Check sheet for the modelled part. Datum: model origin and axes. Units: mm. A direction names the side the tool comes from. Coordinates: 2 decimals unless noted, no trailing zeros. Write each loop counter-clockwise with the first axis right and the second up, starting at its lowest first coordinate (ties: lowest second). Pieces come first, ordered by that corner, then holes. Notation, with made-up numbers: (-14, 40) - (19, 40) arc R20 ccw to (19, 63) - close; hole circle Ø11 at (57.5, 54.5). An arc over 180 degrees is marked (long way). Use one line per item in the form item = value. Start each with the question number.
1. Draft check along Y on faces 1 (the face through (-49.77, 11.85, -10.54)), 2 (the face through (87.24, 4.95, -10.54)), 3 (the face through (217.75, -5.45, -10.54)). Enter one of: +Y half, -Y half, draft (parallel to the pull), parting line (faces both ways), or undercut.
2. Scan lines: line 1 along Y through (x, z) = (197, -9.5); line 2 along Y through (x, z) = (161, -12.1); line 3 along Y through (x, z) = (126.5, -12.05). Record each from-to range of solid material in increasing order.
3. Cross-section at A-A on z = -12.5. Record the boundary of the cut face in (x, y).
4. Cross-section at C-C on y = -34. Record the boundary of the cut face in (x, z).
5. Cross-section at B-B on x = 173. Record the boundary of the cut face in (y, z), then the cut area to 3 significant figures.
6. Go/stop test with flat-tipped pins: pin 1 Ø1.5 at (x, z) = (13.5, -11) entering from -Y; pin 2 Ø1.5 at (y, z) = (4, -8.5) entering from -X; pin 3 Ø2 at (x, z) = (-4, -12) entering from +Y. Record where each tip stops, or that it passes through.
7. Tool access check on faces 4 (the face through (159, -12.5, -11)), 5 (the face through (237.707, 7.5, -10.542)). Record the directions out of +Z, -Z, +X, -X, +Y, -Y that give a thin tool (end or side, any length) a straight path to the whole face; none if there is none.
```python
from build123d import *

# Parameters (mm, degrees)
SKETCH4_R           = 2.55
SKETCH4_R_2         = 2.549999993
SKETCH4_R_3         = 6
BOSS_EXTRUDE1_DEPTH = 6
CUT_EXTRUDE1_DEPTH  = 10


with BuildPart() as part:
    # Sketch4 → Boss-Extrude1 (new body)
    with BuildSketch(Plane.XY.offset(-13.5)):
        with BuildLine():
            Line((197.399795586, 12.5), (89.263654418, 12.5))
            ThreePointArc((89.263654418, 12.5), (87.876262264, 12.337391799), (86.564070557, 11.858381004))
            ThreePointArc((86.564070557, 11.858381004), (21.105246497, -3.69943352), (-44.353577564, 11.858381004))
            ThreePointArc((-44.353577564, 11.858381004), (-49.84201029, 11.812468541), (-52.996718657, 7.321052632))
            ThreePointArc((-52.996718657, 7.321052632), (-26.920402355, -46.233558559), (32.526685027, -42.476637828))
            ThreePointArc((32.526685027, -42.476637828), (74.2820165, -20.197808109), (120.978886956, -12.5))
            Line((120.978886956, -12.5), (197.399795586, -12.5))
            ThreePointArc((197.399795586, -12.5), (199.721224158, -12.282547349), (201.961884602, -11.637755102))
            Line((201.961884602, -11.637755102), (233.980730892, 0.913877551))
            ThreePointArc((233.980730892, 0.913877551), (237.686550892, 7.614285714), (231.790928164, 12.5))
            Line((231.790928164, 12.5), (197.399795586, 12.5))
        make_face()
        with Locations((160.527291291, -6.5)):
            Circle(SKETCH4_R, mode=Mode.SUBTRACT)
        with Locations((89.263654418, 6.5)):
            Circle(SKETCH4_R_2, mode=Mode.SUBTRACT)
        with Locations((21.105246497, -42.553713943)):
            Circle(SKETCH4_R_2, mode=Mode.SUBTRACT)
        with Locations((-47.053161424, 6.5)):
            Circle(SKETCH4_R, mode=Mode.SUBTRACT)
        with Locations((197.399795586, 0)):
            Circle(SKETCH4_R_3, mode=Mode.SUBTRACT)
        with Locations((231.790928164, 6.5)):
            Circle(SKETCH4_R, mode=Mode.SUBTRACT)
    extrude(amount=BOSS_EXTRUDE1_DEPTH)

    # Sketch5 → Cut-Extrude1 (cut)
    with BuildSketch(Plane.XY.offset(-7.5)):
        with BuildLine():
            Line((191.03471214, 1.775352078), (192.679753863, 4.624647922))
            ThreePointArc((192.679753863, 4.624647922), (193.704753863, 6.4), (195.754753863, 6.4))
            Line((195.754753863, 6.4), (199.044837309, 6.4))
            ThreePointArc((199.044837309, 6.4), (201.094837309, 6.4), (202.119837309, 4.624647922))
            Line((202.119837309, 4.624647922), (203.764879032, 1.775352078))
            ThreePointArc((203.764879032, 1.775352078), (204.789879032, 0), (203.764879032, -1.775352078))
            Line((203.764879032, -1.775352078), (202.119837309, -4.624647922))
            ThreePointArc((202.119837309, -4.624647922), (201.094837309, -6.4), (199.044837309, -6.4))
            Line((199.044837309, -6.4), (195.754753863, -6.4))
            ThreePointArc((195.754753863, -6.4), (193.704753863, -6.4), (192.679753863, -4.624647922))
            Line((192.679753863, -4.624647922), (191.03471214, -1.775352078))
            ThreePointArc((191.03471214, -1.775352078), (190.00971214, 0), (191.03471214, 1.775352078))
        make_face()
    extrude(amount=-CUT_EXTRUDE1_DEPTH, mode=Mode.SUBTRACT)


solid = part.part
```
Final values:
q1.face_1 = +Y half
q1.face_2 = undercut
q1.face_3 = -Y half
q2.line_1 = -12.5 to -6.4, 6.4 to 12.5
q2.line_2 = -12.5 to -9.01, -3.99 to 12.5
q2.line_3 = -12.5 to 12.5
q3.outline = (-53, 7.32) arc R53.5 ccw to (32.53, -42.48) arc R145.49 cw to (120.98, -12.5) - (197.4, -12.5) arc R12.5 ccw to (201.96, -11.64) - (233.98, 0.91) arc R6 ccw to (231.79, 12.5) - (89.26, 12.5) arc R6 ccw to (86.56, 11.86) arc R145.49 cw to (-44.35, 11.86) arc R6 ccw to start; hole circle Ø5.1 at (-47.05, 6.5); hole circle Ø5.1 at (21.11, -42.55); hole circle Ø5.1 at (89.26, 6.5); hole circle Ø5.1 at (160.53, -6.5); hole (191.03, -1.78) - (192.68, -4.62) arc R2.05 ccw to (195.75, -6.4) - (199.04, -6.4) arc R2.05 ccw to (202.12, -4.62) - (203.76, -1.78) arc R2.05 ccw to (203.76, 1.78) - (202.12, 4.62) arc R2.05 ccw to (199.04, 6.4) - (195.75, 6.4) arc R2.05 ccw to (192.68, 4.62) - (191.03, 1.78) arc R2.05 ccw to start; hole circle Ø5.1 at (231.79, 6.5)
q4.outline = (-41.31, -13.5) - (44.86, -13.5) - (44.86, -7.5) - (-41.31, -7.5) - close
q5.outline = (-12.5, -13.5) - (12.5, -13.5) - (12.5, -7.5) - (-12.5, -7.5) - close
q5.area = 150 mm²
q6.pin_1 = -51.96
q6.pin_2 = -53.4
q6.pin_3 = -1.34
q7.face_4 = +Z, -Z, +X, -Y
q7.face_5 = +Z, -Z, +X
